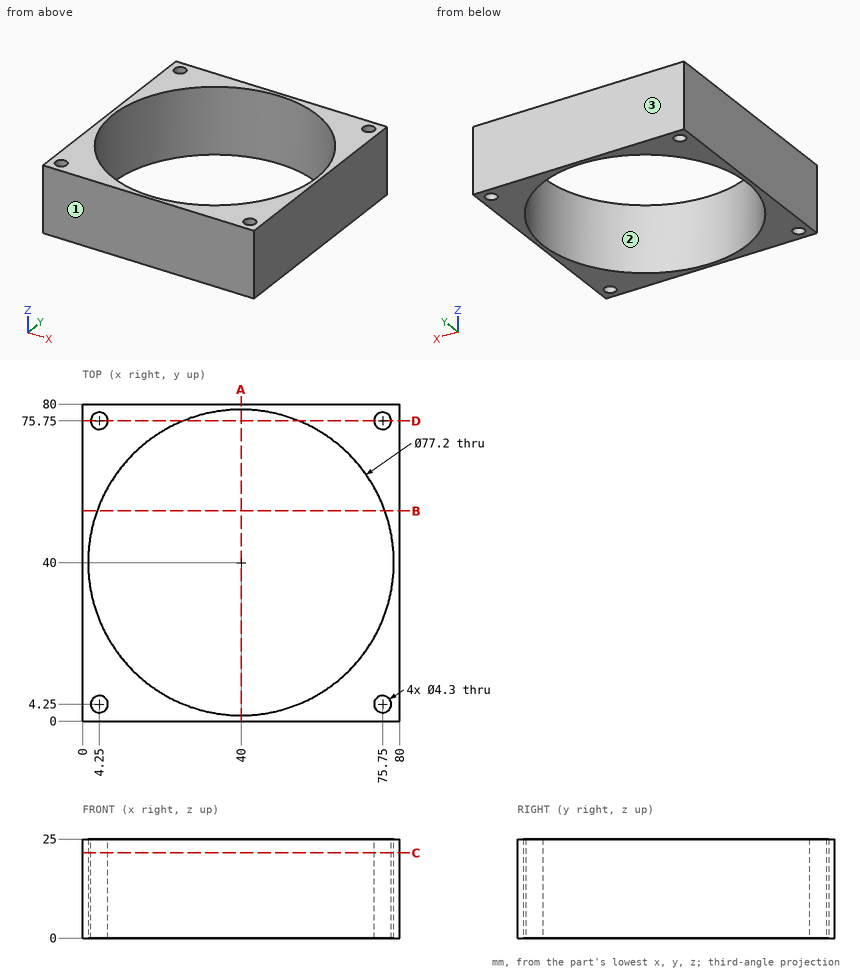
Here's the drawing with two shaded views (mm, measured from the low corner). I have some questions. Coordinates: 2 decimals unless noted, no trailing zeros. Loops run counter-clockwise (first coordinate to the right, second up) from the corner with the lowest first, then second, coordinate; pieces in that order, holes last. Notation, with made-up numbers: (-6, -7) -> (17, -7) arc R24 cw to (17, 19) -> close; hole circle Ø2 at (87.5, -32.5). An arc over 180 degrees is marked (long way). Answer in a Markdown table with one row per item.
(1) Imagine slicing it at A-A (x = 40). List the corners of the cut face in (y, z) for me.
Results found:
| item | result |
|---|---|
| outline | (0, 0) -> (1.4, 0) -> (1.4, 25) -> (0, 25) -> close; (78.6, 0) -> (80, 0) -> (80, 25) -> (78.6, 25) -> close |
(2) Imagine slicing it at D-D (y = 75.75). List the corners of the cut face in (x, z) for me.
Results found:
| item | result |
|---|---|
| outline | (0, 0) -> (2.1, 0) -> (2.1, 25) -> (0, 25) -> close; (6.4, 0) -> (25.44, 0) -> (25.44, 25) -> (6.4, 25) -> close; (54.56, 0) -> (73.6, 0) -> (73.6, 25) -> (54.56, 25) -> close; (77.9, 0) -> (80, 0) -> (80, 25) -> (77.9, 25) -> close |
(3) Thinking about a two-plate mould opening in Y: for the marked faces 1, 2 and 3, which applies, released by +Y, released by -Y, zero draft, split by the parting line, or undercut?
Results found:
| item | result |
|---|---|
| face 1 | released by -Y |
| face 2 | undercut |
| face 3 | released by +Y |
(4) If I drill on probe 1 along Y at (x, z) = (40, 10); probe 2 along Y at (x, z) = (24, 15); probe 3 along X at (y, z) = (15, 9), over which ranges is the centre line in solid material (lowest first)?
Results found:
| item | result |
|---|---|
| probe 1 | y = 0 to 1.4, 78.6 to 80 |
| probe 2 | y = 0 to 4.87, 75.13 to 80 |
| probe 3 | x = 0 to 10.59, 69.41 to 80 |
(5) Imagine slicing it at B-B (y = 53). List the corners of the cut face in (x, z) for me.
Results found:
| item | result |
|---|---|
| outline | (0, 0) -> (3.65, 0) -> (3.65, 25) -> (0, 25) -> close; (76.35, 0) -> (80, 0) -> (80, 25) -> (76.35, 25) -> close |
(6) Imagine slicing it at C-C (z = 21.5). List the corners of the cut face in (x, y) for me, plus the area to 3 significant figures.
Results found:
| item | result |
|---|---|
| outline | (0, 0) -> (80, 0) -> (80, 80) -> (0, 80) -> close; hole circle Ø77.2 at (40, 40); hole circle Ø4.3 at (4.25, 4.25); hole circle Ø4.3 at (4.25, 75.75); hole circle Ø4.3 at (75.75, 4.25); hole circle Ø4.3 at (75.75, 75.75) |
| area | 1,660 mm^2 |
(7) Will this pin go through, and if not, where does the flat tip stop? pin 1 Ø3.5 at (x, y) = (75.75, 75.75) entering from -Z.
Results found:
| item | result |
|---|---|
| pin 1 | passes through |
